Model file for the job. Use its own axes, mm. A direction names the side the tool comes from. Round coordinates to 2 decimals unless told otherwise and drop trailing zeros. Write each loop counter-clockwise with the first axis right and the second up, starting at its lowest first coordinate (ties: lowest second). Pieces come first, ordered by that corner, then holes. Notation, with made-up numbers: (26.5, 43.25) - (64.5, 43.25) arc R21 cw to (64.5, 56.25) - close; hole circle Ø3 at (43, -39.75). An arc over 180 degrees is marked (long way). One line per item, written item: value.
from build123d import *

# Parameters (mm, degrees)
SKETCH_W     = 30
SKETCH_H     = 42
PAD_DEPTH    = 5
SKETCH001_R  = 2.55
PAD001_DEPTH = 20
SKETCH002_W  = 42
SKETCH002_H  = 3
POCKET_DEPTH = 30.001


with BuildPart() as part:
    # Sketch → Pad (new body)
    with BuildSketch(Plane.XY):
        Rectangle(SKETCH_W, SKETCH_H)
    extrude(amount=PAD_DEPTH)

    # Sketch001 (on Face3 of Pad) → Pad001 (join)
    with BuildSketch(Plane.XZ.offset(21)):
        with BuildLine():
            ThreePointArc((5, 5), (0, 10), (-5, 5))
            Line((-5, 5), (-5, 0))
            Line((-5, 0), (5, 0))
            Line((5, 0), (5, 5))
        make_face()
        with Locations((0, 5)):
            Circle(SKETCH001_R, mode=Mode.SUBTRACT)
    extrude(amount=PAD001_DEPTH)

    # Sketch002 (on Face2 of Pad001) → Pocket (cut, through all)
    with BuildSketch(Plane(origin=(-15, 0, 0), x_dir=(0, -1, 0), z_dir=(-1, 0, 0))):
        with Locations((0, 3.5)):
            Rectangle(SKETCH002_W, SKETCH002_H)
    extrude(amount=-POCKET_DEPTH, mode=Mode.SUBTRACT)


solid = part.part
1. Band-saw the part on C-C on y = -24. Write the cut outline in (x, z).
Report:
outline: (-5, 0) - (5, 0) - (5, 5) arc R5 ccw to (-5, 5) - close; hole circle Ø5.1 at (0, 5)
2. Tool access for faces 1 (the face through (10, -21, 1)), 2 (the face through (-10, -21, 1)), 3 (the face through (-15, 0, 1)), 4 (the face through (0, 21, 1)), 5 (the face through (0, 0, 2)): list every direction of +Z, -Z, +X, -X, +Y, -Y with a clear straight run to the whole face (end or side of a thin tool).
Report:
face 1: +Z, -Z, +X, -Y
face 2: +Z, -Z, -X, -Y
face 3: +Z, -Z, -X, +Y, -Y
face 4: +Z, -Z, +X, -X, +Y
face 5: +Z, +X, -X, +Y
3. Drop flat-ended pins along their axis: pin 1 (1 mm diameter, centred on x = -9.5, z = 1, fed in from -Y); pin 2 (10 mm diameter, centred on x = -3.5, y = -18, fed in from +Z); pin 3 (1.5 mm diameter, centred on y = -27.5, z = 7.5, fed in from +X); pin 4 (1 mm diameter, centred on y = -31.5, z = 2.5, fed in from -X). Give the stop position or say it passes through.
Report:
pin 1: y = -21
pin 2: z = 10
pin 3: x = 4.68
pin 4: x = -5
4. Band-saw the part on D-D on x = -3.5. Write the cut outline in (y, z), plus the area to 3 significant figures.
Report:
outline: (-41, 0) - (21, 0) - (21, 2) - (-21, 2) - (-21, 8.57) - (-41, 8.57) - close
area: 255 mm²
5. Wall check: probe 1 along Z at (x, y) = (0, -27.5); probe 2 along Z at (x, y) = (9.75, 13); probe 3 along X at (y, z) = (-27.5, 2). Give the ranges that are in metal, low to high. Write a range as [from, to].
Report:
probe 1: [0, 2.45], [7.55, 10]
probe 2: [0, 2]
probe 3: [-5, 5]
6. Mould opens along Z. For faces 6 (the face through (0, -31, 10)), 7 (the face through (-5, -31, 3)), 8 (the face through (1.37, -30.86, 7.15)) say: released by +Z, released by -Z, zero draft, split by the parting line, or undercut.
Report:
face 6: released by +Z
face 7: zero draft
face 8: undercut
7. Band-saw the part on B-B on z = 6. Write the cut outline in (x, y).
Report:
outline: (-4.9, -41) - (-2.35, -41) - (-2.35, -21) - (-4.9, -21) - close; (2.35, -41) - (4.9, -41) - (4.9, -21) - (2.35, -21) - close
8. Band-saw the part on A-A on x = 0. Write the cut outline in (y, z).
Report:
outline: (-41, 0) - (21, 0) - (21, 2) - (-21, 2) - (-21, 2.45) - (-41, 2.45) - close; (-41, 7.55) - (-21, 7.55) - (-21, 10) - (-41, 10) - close
